```python
from build123d import *

# Parameters (mm, degrees)
SKETCH1_R           = 4.7625
SKETCH1_R_2         = 2.0193
BOSS_EXTRUDE1_DEPTH = 103.251
SKETCH2_R           = 4.7625
BOSS_EXTRUDE2_DEPTH = 103.251


with BuildPart() as part:
    # Sketch1 → Boss-Extrude1 (new body)
    with BuildSketch(Plane.XY):
        Circle(SKETCH1_R)
        Circle(SKETCH1_R_2, mode=Mode.SUBTRACT)
    extrude(amount=BOSS_EXTRUDE1_DEPTH)

    # Sketch2 → Boss-Extrude2 (add, through all)
    with BuildSketch(Plane.XY.offset(103.251)):
        Polygon((7.332348419, 0), (3.666174209, 6.35), (-3.666174209, 6.35), (-7.332348419, 0), (-3.666174209, -6.35), (3.666174209, -6.35), align=None)
        Circle(SKETCH2_R, mode=Mode.SUBTRACT)
    extrude(amount=-BOSS_EXTRUDE2_DEPTH)


solid = part.part
```
The listing builds one solid part. Answer for the finished solid, in the listing's coordinates (mm). Round coordinates to 2 decimals unless told otherwise and drop trailing zeros. Loops run counter-clockwise (first coordinate to the right, second up) from the corner with the lowest first, then second, coordinate; pieces in that order, holes last.
Q1. Find the intervals of material crossed by line 1 (Y direction, x = 0, z = 43.5); line 2 (Y direction, x = 0.75, z = 78); line 3 (X direction, y = -0.75, z = 85.5), in increasing order.
Q2. Section B-B, the plane x = 0 is taken. Determine the outline of the cut face in (y, z).
Q3. Section A-A, the plane z = 57 is taken. Determine the outline of the cut face in (x, y), then the cut area to 3 significant figures.
Q4. Given pin 1 Ø6 at (y, z) = (-4, 78.5) entering from -X (3 decimals); pin 2 Ø4 at (y, z) = (3, 52.5) entering from +X (3 decimals); pin 3 Ø3 at (y, z) = (4.5, 55) entering from +X, each flat-ended and moving along its own axis, determine where each tip first touches the part or whether it passes through.
Q5. Section C-C, the plane y = -4.75 is taken. Determine the outline of the cut face in (x, z), then the cut area to 3 significant figures.
Q6. For a pull along X with two mould halves and no side action, classify faces 1 (the face through (5.525, 3.131, 52.348)), 2 (the face through (2, 2, 103.251)), 3 (the face through (-5.525, -3.131, 52.348)), 4 (the face through (1.926, 0.607, 50.903)) as released by +X, released by -X, zero draft, split by the parting line, or undercut.
Q7. Section D-D, the plane x = -5.25 is taken. Determine the outline of the cut face in (y, z), then the cut area to 3 significant figures.
Completed:
1. line 1: y = -6.35 to -2.02, 2.02 to 6.35
1. line 2: y = -6.35 to -1.87, 1.87 to 6.35
1. line 3: x = -6.9 to -1.87, 1.87 to 6.9
2. outline: (-6.35, 0) - (-2.02, 0) - (-2.02, 103.25) - (-6.35, 103.25) - close; (2.02, 0) - (6.35, 0) - (6.35, 103.25) - (2.02, 103.25) - close
3. outline: (-7.33, 0) - (-3.67, -6.35) - (3.67, -6.35) - (7.33, 0) - (3.67, 6.35) - (-3.67, 6.35) - close; hole circle Ø4.04 at (0, 0)
3. area: 127 mm2
4. pin 1: stops at x = -6.755
4. pin 2: stops at x = 6.755
4. pin 3: stops at x = 5.6
5. outline: (-4.59, 0) - (4.59, 0) - (4.59, 103.25) - (-4.59, 103.25) - close
5. area: 948 mm2
6. face 1: released by +X
6. face 2: zero draft
6. face 3: released by -X
6. face 4: undercut
7. outline: (-3.61, 0) - (3.61, 0) - (3.61, 103.25) - (-3.61, 103.25) - close
7. area: 745 mm2
